Job drawing, mm, ordinate dimensions from the low corner. One solid piece. A direction names the side the tool comes from. Give positions to 0.01 mm unless a question says otherwise; leave off trailing zeros. Write each loop counter-clockwise with the first axis right and the second up, starting at its lowest first coordinate (ties: lowest second). Pieces come first, ordered by that corner, then holes. Notation, with made-up numbers: M 80,22 L 111,22 A12 cw 111,31 Z; hole C -32.5,-13.5 d5. An arc over 180 degrees is marked long. Use CSV: the item, a comma, the result in double quotes. Start each with the question number.
Item 1: Cut at A-A (x = 10). List the corners of the cut face in (y, z).
Item 2: Mould opens along Z. For the marked faces 3, 4, 5 and 6 say: released by +Z, released by -Z, zero draft, split by the parting line, or undercut.
Item 3: Cut at C-C (z = 4.75). List the corners of the cut face in (x, y), then the cut area to 3 significant figures.
Item 4: Cut at B-B (y = 0.85). List the corners of the cut face in (x, z).
Item 5: Drill centre lines: line 1 (Z direction, x = 10, y = 0.8); line 2 (X direction, y = 1.25, z = 5.25); line 3 (X direction, y = 2.45, z = 6.25). Where is each one in solid material? Low to high. Write a range as [from, to].
Item 6: Which spindle directions (+Z, -Z, +X, -X, +Y, -Y) get a long thin tool onto all of the face, cutting with end or side? Do the marked faces 1 and 2. Say none if no direction does.
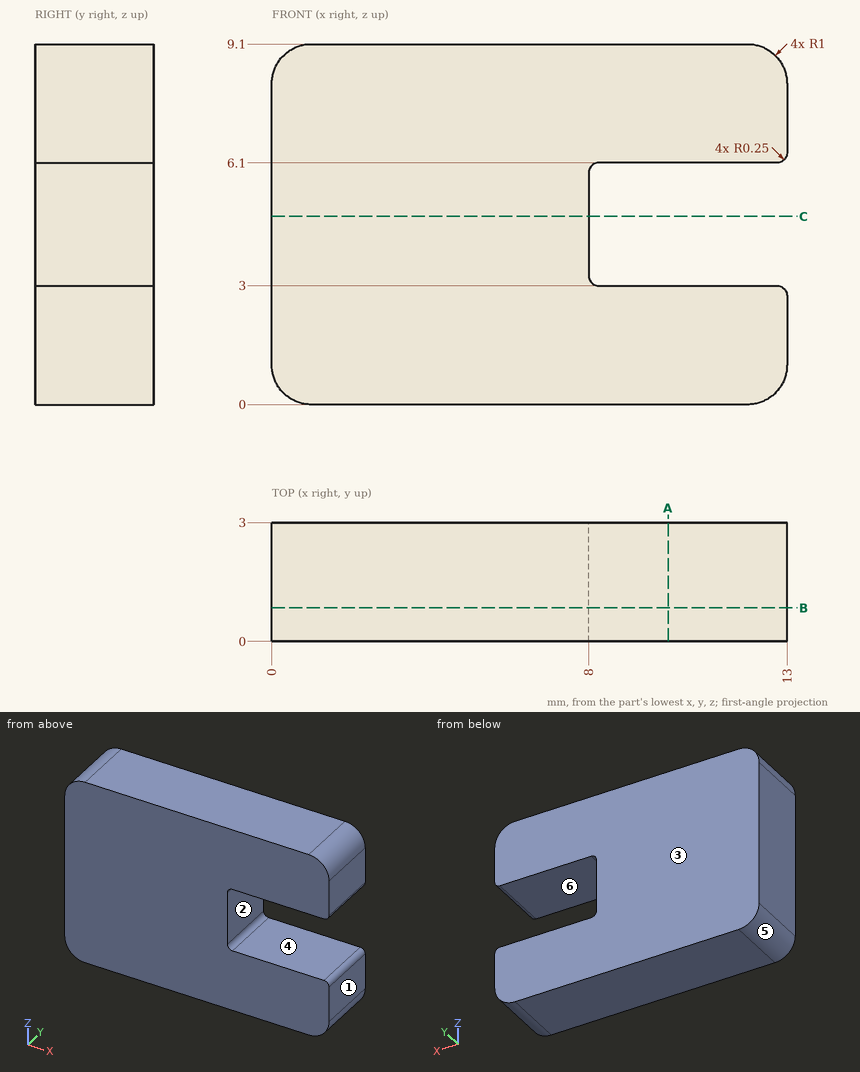
Worked answers:
1,outline,"M 0,0 L 3,0 L 3,3 L 0,3 Z; M 0,6.1 L 3,6.1 L 3,9.1 L 0,9.1 Z"
2,face 3,"zero draft"
2,face 4,"undercut"
2,face 5,"released by -Z"
2,face 6,"undercut"
3,outline,"M 0,0 L 8,0 L 8,3 L 0,3 Z"
3,area,"24.0 mm^2"
4,outline,"M 0,1 A1 ccw 1,0 L 12,0 A1 ccw 13,1 L 13,2.75 A0.25 ccw 12.75,3 L 8.25,3 A0.25 cw 8,3.25 L 8,5.85 A0.25 cw 8.25,6.1 L 12.75,6.1 A0.25 ccw 13,6.35 L 13,8.1 A1 ccw 12,9.1 L 1,9.1 A1 ccw 0,8.1 Z"
5,line 1,"z = [0, 3], [6.1, 9.1]"
5,line 2,"x = [0, 8]"
5,line 3,"x = [0, 12.98]"
6,face 1,"+Z, -Z, +X, +Y, -Y"
6,face 2,"+X, +Y, -Y"
